Here's the drawing with two shaded views (mm, measured from the low corner). I have some questions. Coordinates: 2 decimals unless noted, no trailing zeros. Write each loop counter-clockwise with the first axis right and the second up, starting at its lowest first coordinate (ties: lowest second). Pieces come first, ordered by that corner, then holes. Notation, with made-up numbers: (-3, 89.25) -> (11, 89.25) arc R37 cw to (11, 125.25) -> close; hole circle Ø3 at (-38.75, -22). An arc over 180 degrees is marked (long way). Use a Markdown table: item, result. Add a question column.
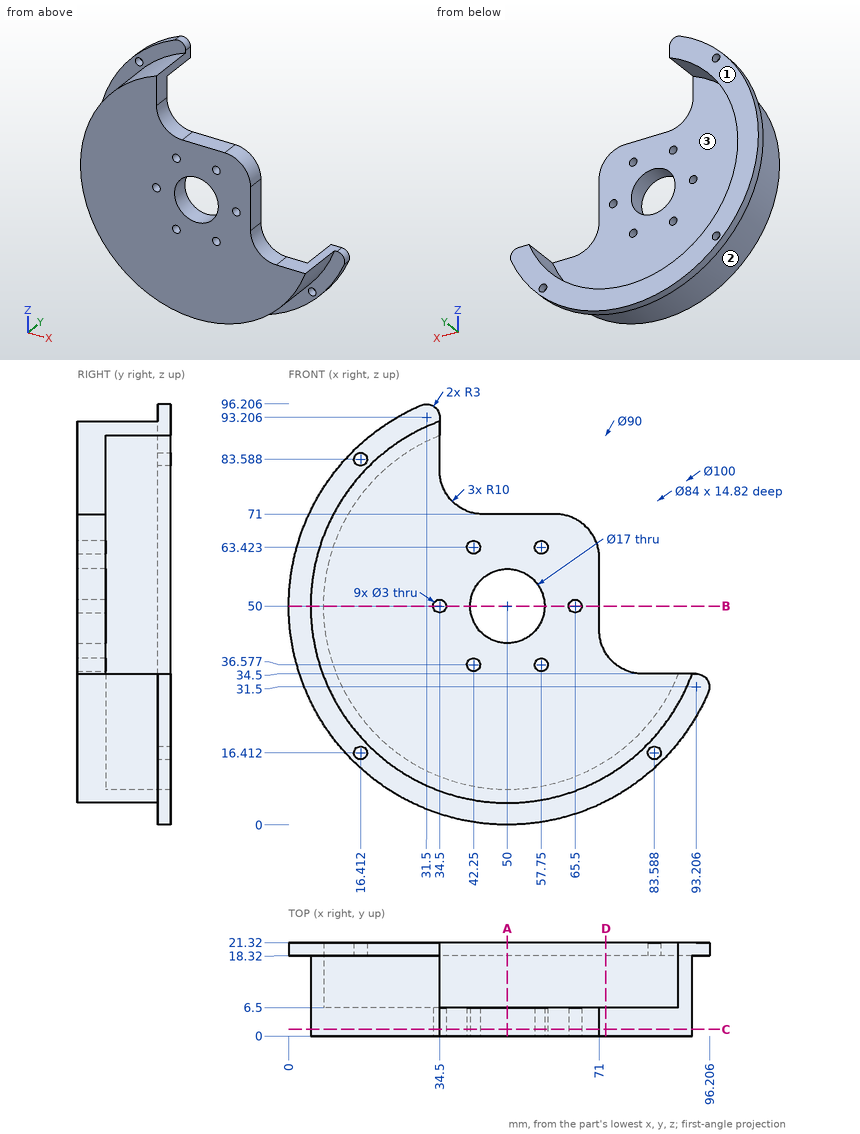
Q1. Suppose I cut it at D-D, the plane x = 72.5. Write out the boundary of the cut face in (y, z) (1 decimal), and give its area (3 significant figures).
Q2. Will these pins go through, and if not, where does the flat tip stop? pin 1 (4 mm diameter, centred on x = 16.41, z = 83.59, fed in from -Y); pin 2 (10 mm diameter, centred on x = 49, y = 13.5, fed in from +Z); pin 3 (5 mm diameter, centred on x = 75, y = 17.5, fed in from -Z); pin 4 (3.5 mm diameter, centred on x = 83.59, z = 16.41, fed in from +Y).
Q3. Suppose I cut it at C-C, the plane y = 1.5. Write out the boundary of the cut face in (x, z), and give its area (3 significant figures).
Q4. Suppose I cut it at B-B, the plane z = 50. Write out the boundary of the cut face in (x, y).
Q5. Suppose I cut it at A-A, the plane x = 50. Write out the boundary of the cut face in (y, z), and give its area (3 significant figures).
Q6. Please list where these lines run through material, in increasing order: line 1 (X direction, y = 3.25, z = 50); line 2 (Z direction, x = 57.75, y = 3.75) (1 decimal); line 3 (Y direction, x = 39.5, z = 68).
Q7. Thinking about a two-plate mould opening in X: for the marked faces 1, 2 and 3, which applies, released by +X, released by -X, zero draft, split by the parting line, or undercut?
Answer key:
| question | item | result |
|---|---|---|
| 1 | outline | (0, 11) -> (18.3, 11) -> (18.3, 5.3) -> (21.3, 5.3) -> (21.3, 14.5) -> (6.5, 14.5) -> (6.5, 39.2) -> (0, 39.2) -> close |
| 1 | area | 252 mm^2 |
| 2 | pin 1 | stops at y = 18.32 |
| 2 | pin 2 | stops at z = 8.43 |
| 2 | pin 3 | stops at z = 5.42 |
| 2 | pin 4 | stops at y = 21.32 |
| 3 | outline | (34.5, 81) -> (34.5, 92.25) arc R45 ccw (long way) to (92.25, 34.5) -> (81, 34.5) arc R10 cw to (71, 44.5) -> (71, 61) arc R10 ccw to (61, 71) -> (44.5, 71) arc R10 cw to start; hole circle Ø3 at (34.5, 50); hole circle Ø3 at (42.25, 36.58); hole circle Ø3 at (42.25, 63.42); hole circle Ø17 at (50, 50); hole circle Ø3 at (57.75, 36.58); hole circle Ø3 at (57.75, 63.42); hole circle Ø3 at (65.5, 50) |
| 3 | area | 4,250 mm^2 |
| 4 | outline | (0, 18.32) -> (5, 18.32) -> (5, 0) -> (33, 0) -> (33, 6.5) -> (8, 6.5) -> (8, 21.32) -> (0, 21.32) -> close; (36, 0) -> (41.5, 0) -> (41.5, 6.5) -> (36, 6.5) -> close; (58.5, 0) -> (64, 0) -> (64, 6.5) -> (58.5, 6.5) -> close; (67, 0) -> (71, 0) -> (71, 6.5) -> (67, 6.5) -> close |
| 5 | outline | (0, 5) -> (18.32, 5) -> (18.32, 0) -> (21.32, 0) -> (21.32, 8) -> (6.5, 8) -> (6.5, 41.5) -> (0, 41.5) -> close; (0, 58.5) -> (6.5, 58.5) -> (6.5, 71) -> (0, 71) -> close |
| 5 | area | 378 mm^2 |
| 6 | line 1 | x = 5 to 33, 36 to 41.5, 58.5 to 64, 67 to 71 |
| 6 | line 2 | z = 5.7 to 35.1, 38.1 to 46.5, 53.5 to 61.9, 64.9 to 71 |
| 6 | line 3 | y = 0 to 6.5 |
| 7 | face 1 | zero draft |
| 7 | face 2 | split by the parting line |
| 7 | face 3 | undercut |
